Check sheet for the modelled part. Datum: model origin and axes. Units: mm. Face numbers are marked on the shaded views. A direction names the side the tool comes from. Give positions to 0.01 mm unless a question says otherwise; leave off trailing zeros. Order: outer loops, then holes, each group sorted by start corner. A loop starts at its lowest first (then second) coordinate and runs counter-clockwise, first axis right, second up.
Item 1: Material ranges on line 1 along Y through (x, z) = (0, 1.95); line 2 along Z through (x, y) = (2.5, -2.5); line 3 along Y through (x, z) = (0, 1.6), recorded low to high.
Item 2: Sectioned sample at A-A on x = 0. Record the boundary of the cut face in (y, z).
Item 3: Sectioned sample at C-C on z = 1. Record the boundary of the cut face in (x, y), and give its area (3 significant figures).
Item 4: Access from +Z, -Z, +X, -X, +Y, -Y to the whole of each face (thin tool, end or side, straight path). Record for the marked faces 1 and 2.
Item 5: Release check for a two-part mould opening along X. For the marked faces 3 and 4 record: released by +X, released by -X, zero draft, split by the parting line, or undercut.
Item 6: Sectioned sample at D-D on x = -2.75. Record the boundary of the cut face in (y, z).
from build123d import *

# Parameters (mm, degrees)
SKETCH1_R           = 5
SKETCH1_R_2         = 2.5
BOSS_EXTRUDE1_DEPTH = 2
SKETCH2_R           = 4.5
SKETCH2_R_2         = 3
CUT_EXTRUDE1_DEPTH  = 0.1


with BuildPart() as part:
    # Sketch1 → Boss-Extrude1 (new, symmetric)
    with BuildSketch(Plane.XY):
        Circle(SKETCH1_R)
        Circle(SKETCH1_R_2, mode=Mode.SUBTRACT)
    extrude(amount=BOSS_EXTRUDE1_DEPTH, both=True)

    # Sketch2 → Cut-Extrude1 (cut)
    with BuildSketch(Plane.XY.offset(2)):
        Circle(SKETCH2_R)
        Circle(SKETCH2_R_2, mode=Mode.SUBTRACT)
    cut_extrude1 = extrude(amount=-CUT_EXTRUDE1_DEPTH, mode=Mode.SUBTRACT)

    # Mirror1: Cut-Extrude1 across plane
    add(cut_extrude1.mirror(Plane.XY), mode=Mode.SUBTRACT)


solid = part.part
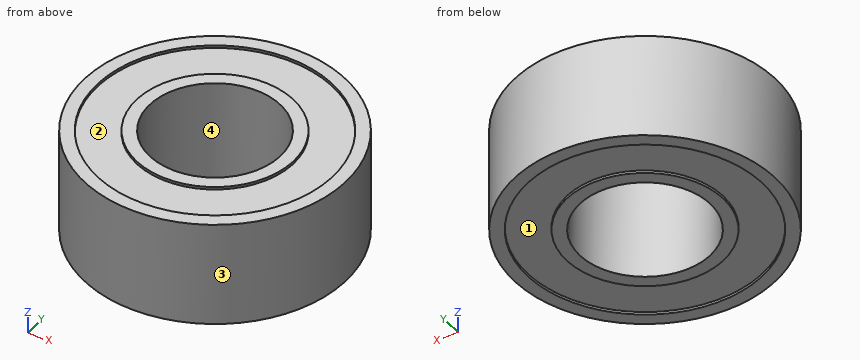
Report:
1. line 1: y = -5 to -4.5, -3 to -2.5, 2.5 to 3, 4.5 to 5
1. line 2: z = -1.9 to 1.9
1. line 3: y = -5 to -2.5, 2.5 to 5
2. outline: (-5, -2) - (-4.5, -2) - (-4.5, -1.9) - (-3, -1.9) - (-3, -2) - (-2.5, -2) - (-2.5, 2) - (-3, 2) - (-3, 1.9) - (-4.5, 1.9) - (-4.5, 2) - (-5, 2) - close; (2.5, -2) - (3, -2) - (3, -1.9) - (4.5, -1.9) - (4.5, -2) - (5, -2) - (5, 2) - (4.5, 2) - (4.5, 1.9) - (3, 1.9) - (3, 2) - (2.5, 2) - close
3. outline: circle Ø10 at (0, 0); hole circle Ø5 at (0, 0)
3. area: 58.9 mm2
4. face 1: -Z
4. face 2: +Z
5. face 3: split by the parting line
5. face 4: undercut
6. outline: (-4.18, -2) - (-3.56, -2) - (-3.56, -1.9) - (-1.2, -1.9) - (-1.2, -2) - (1.2, -2) - (1.2, -1.9) - (3.56, -1.9) - (3.56, -2) - (4.18, -2) - (4.18, 2) - (3.56, 2) - (3.56, 1.9) - (1.2, 1.9) - (1.2, 2) - (-1.2, 2) - (-1.2, 1.9) - (-3.56, 1.9) - (-3.56, 2) - (-4.18, 2) - close
